Design review of the part built by this model. Coordinates are the model's own, in mm. A direction names the side the tool comes from. Coordinates: 2 decimals unless noted, no trailing zeros. Write each loop counter-clockwise with the first axis right and the second up, starting at its lowest first coordinate (ties: lowest second). Pieces come first, ordered by that corner, then holes. Notation, with made-up numbers: (42, -21.75) - (72, -21.75) arc R20 ccw to (72, -12.75) - close; hole circle Ø10 at (45.25, 79.5). An arc over 180 degrees is marked (long way). Use a Markdown table: item, result.
from build123d import *

# Parameters (mm, degrees)
ESQUISSE1_W             = 218
ESQUISSE1_H             = 80
ESQUISSE1_W_2           = 208
ESQUISSE1_H_2           = 70
BOSS_EXTRU_1_DEPTH      = 16.5
ESQUISSE2_W             = 15
ESQUISSE2_H             = 80
ESQUISSE2_R             = 3.25
BOSS_EXTRU_2_DEPTH      = 2.45
ESQUISSE3_W             = 22
ESQUISSE3_H             = 5
ENL_V_MAT_EXTRU_1_DEPTH = 16.5
ESQUISSE4_W             = 15
ESQUISSE4_H             = 70
ESQUISSE4_R             = 1.7
BOSS_EXTRU_3_DEPTH      = 3
CONG_1_R                = 20
ESQUISSE7_W             = 22
ESQUISSE7_H             = 5
BOSS_EXTRU_5_DEPTH      = 8
ESQUISSE8_W             = 52.75
ESQUISSE8_H             = 5
ESQUISSE8_W_2           = 24.75
ESQUISSE8_W_3           = 99.5
BOSS_EXTRU_6_DEPTH      = 2.45


with BuildPart() as part:
    # Esquisse1 → Boss.-Extru.1 (new body)
    with BuildSketch(Plane(origin=(0, 0, 0), x_dir=(1, 0, 0), z_dir=(0, 0.342020143, 0.939692621))):
        Rectangle(ESQUISSE1_W, ESQUISSE1_H)
        Rectangle(ESQUISSE1_W_2, ESQUISSE1_H_2, mode=Mode.SUBTRACT)
    extrude(amount=BOSS_EXTRU_1_DEPTH)

    # Esquisse2 → Boss.-Extru.2 (add)
    with BuildSketch(Plane(origin=(0, 0, 0), x_dir=(-1, 0, 0), z_dir=(0, -0.342020143, -0.939692621))):
        with Locations((-45.25, 0)):
            Rectangle(ESQUISSE2_W, ESQUISSE2_H)
        with Locations((-45.25, 29.75)):
            Circle(ESQUISSE2_R, mode=Mode.SUBTRACT)
        with Locations((-45.25, -29.75)):
            Circle(ESQUISSE2_R, mode=Mode.SUBTRACT)
        with Locations((69.25, 0)):
            Rectangle(ESQUISSE2_W, ESQUISSE2_H)
        with Locations((69.25, 29.75)):
            Circle(ESQUISSE2_R, mode=Mode.SUBTRACT)
        with Locations((69.25, -29.75)):
            Circle(ESQUISSE2_R, mode=Mode.SUBTRACT)
    extrude(amount=BOSS_EXTRU_2_DEPTH)

    # Esquisse3 → Enlèv. mat.-Extru.1 (cut)
    with BuildSketch(Plane(origin=(0, 5.643332365, 15.504928243), x_dir=(1, 0, 0), z_dir=(0, 0.342020143, 0.939692621))):
        with Locations((2, -37.5)):
            Rectangle(ESQUISSE3_W, ESQUISSE3_H)
    extrude(amount=-ENL_V_MAT_EXTRU_1_DEPTH, mode=Mode.SUBTRACT)

    # Esquisse4 → Boss.-Extru.3 (add)
    with BuildSketch(Plane(origin=(0, 0, 0), x_dir=(1, 0, 0), z_dir=(0, 0.342020143, 0.939692621))):
        with Locations((45.25, 0)):
            Rectangle(ESQUISSE4_W, ESQUISSE4_H)
        with Locations((45.25, -29.75)):
            Circle(ESQUISSE4_R, mode=Mode.SUBTRACT)
        with Locations((45.25, 29.75)):
            Circle(ESQUISSE4_R, mode=Mode.SUBTRACT)
        with Locations((-69.25, 0)):
            Rectangle(ESQUISSE4_W, ESQUISSE4_H)
        with Locations((-69.25, 29.75)):
            Circle(ESQUISSE4_R, mode=Mode.SUBTRACT)
        with Locations((-69.25, -29.75)):
            Circle(ESQUISSE4_R, mode=Mode.SUBTRACT)
    extrude(amount=BOSS_EXTRU_3_DEPTH)

    # Congé1
    cong_1_edges = [part.edges().sort_by_distance(p)[0] for p in [
        (52.75, -32.376211513, 13.380243948),
        (52.75, 33.402271942, -10.561166085),
        (-76.75, 33.402271942, -10.561166085),
        (-76.75, -32.376211513, 13.380243948),
    ]]
    fillet(cong_1_edges, radius=CONG_1_R)

    # Esquisse7 → Boss.-Extru.5 (add)
    with BuildSketch(Plane(origin=(0, 5.643332365, 15.504928243), x_dir=(1, 0, 0), z_dir=(0, 0.342020143, 0.939692621))):
        with Locations((2, -37.5)):
            Rectangle(ESQUISSE7_W, ESQUISSE7_H)
    extrude(amount=-BOSS_EXTRU_5_DEPTH)

    # Esquisse8 → Boss.-Extru.6 (add)
    with BuildSketch(Plane(origin=(0, 0, 0), x_dir=(-1, 0, 0), z_dir=(0, -0.342020143, -0.939692621))):
        with BuildLine():
            Line((76.75, -15), (76.75, -40))
            Line((76.75, -40), (109, -40))
            Line((109, -40), (109, 40))
            Line((109, 40), (76.75, 40))
            Line((76.75, 40), (76.75, 15))
            ThreePointArc((76.75, 15), (82.607864376, 29.142135624), (96.75, 35))
            Line((96.75, 35), (104, 35))
            Line((104, 35), (104, -35))
            Line((104, -35), (96.75, -35))
            ThreePointArc((96.75, -35), (82.607864376, -29.142135624), (76.75, -15))
        make_face()
        with BuildLine():
            Line((-52.75, 15), (-52.75, 40))
            Line((-52.75, 40), (-109, 40))
            Line((-109, 40), (-109, -40))
            Line((-109, -40), (-52.75, -40))
            Line((-52.75, -40), (-52.75, -15))
            ThreePointArc((-52.75, -15), (-58.607864376, -29.142135624), (-72.75, -35))
            Line((-72.75, -35), (-104, -35))
            Line((-104, -35), (-104, 35))
            Line((-104, 35), (-72.75, 35))
            ThreePointArc((-72.75, 35), (-58.607864376, 29.142135624), (-52.75, 15))
        make_face()
        with Locations((35.375, -37.5)):
            Rectangle(ESQUISSE8_W, ESQUISSE8_H)
        with Locations((-25.375, -37.5)):
            Rectangle(ESQUISSE8_W_2, ESQUISSE8_H)
        with Locations((12, 37.5)):
            Rectangle(ESQUISSE8_W_3, ESQUISSE8_H)
    extrude(amount=BOSS_EXTRU_6_DEPTH)


solid = part.part
(1) Take a section at C-C on z = 18. Write out the cut boundary in (x, y), and give its area (3 significant figures).
Determined:
| item | result |
|---|---|
| outline | (-109, -36.02) - (-9, -36.02) - (-9, -30.69) - (-104, -30.69) - (-104, -1.21) - (-109, -1.21) - close; (13, -36.02) - (109, -36.02) - (109, -1.21) - (104, -1.21) - (104, -30.69) - (13, -30.69) - close |
| area | 1,340 mm2 |
(2) Take a section at A-A on x = -41. Write out the cut boundary in (y, z), and give its area (4 significant figures).
Determined:
| item | result |
|---|---|
| outline | (-38.43, 11.38) - (-33.73, 9.67) - (-27.25, 27.48) - (-31.94, 29.19) - close; (32.05, -14.27) - (36.75, -15.98) - (43.23, 1.82) - (38.53, 3.53) - close |
| area | 189.5 mm2 |
(3) Draft analysis for pull direction Z (two halves, no side actions). For faces 1 (the flat face through (-1.46, -29.72, 20.68)), 2 (the flat face through (-76.75, 0, 0)), 3 (the flat face through (1.456, 36.057, -3.266)), state which applies: +Z half, -Z half, draft (parallel to the pull), parting line (faces both ways), or undercut.
Determined:
| item | result |
|---|---|
| face 1 | undercut |
| face 2 | draft |
| face 3 | +Z half |
(4) Take a section at B-B on y = 11. Write out the cut boundary in (x, z), and give its area (3 significant figures).
Determined:
| item | result |
|---|---|
| outline | (-109, -6.61) - (-104, -6.61) - (-104, 13.56) - (-109, 13.56) - close; (-76.75, -6.61) - (-61.75, -6.61) - (-61.75, -0.81) - (-76.75, -0.81) - close; (37.75, -6.61) - (52.75, -6.61) - (52.75, -0.81) - (37.75, -0.81) - close; (104, -6.61) - (109, -6.61) - (109, 13.56) - (104, 13.56) - close |
| area | 376 mm2 |
(5) Take a section at D-D on x = 0. Write out the cut boundary in (y, z).
Determined:
| item | result |
|---|---|
| outline | (-34.68, 21.67) - (-29.98, 19.96) - (-27.25, 27.48) - (-31.94, 29.19) - close; (32.05, -14.27) - (36.75, -15.98) - (43.23, 1.82) - (38.53, 3.53) - close |
(6) For pin 1 (8 mm diameter, centred on x = 80.5, z = 22.5, fed in from +Y); pin 2 (5 mm diameter, centred on x = 41.5, y = -22.5, fed in from +Z); pin 3 (3 mm diameter, centred on x = -63, z = 2.5, fed in from +Y), all flat-tipped, find the tip position at first contact; note any pin that passes through.
Determined:
| item | result |
|---|---|
| pin 1 | y = -27.6 |
| pin 2 | z = 12.29 |
| pin 3 | y = 43.23 |
(7) Machinability: for faces 4 (the flat face through (0.51, 35.53, -15.54)), 5 (the flat face through (46.649, 26.641, -9.697)), 6 (the flat face through (1.8, -32.3, 20.8)), 7 (the flat face through (52.75, 0, 0)), which of the approach directions +Z, -Z, +X, -X, +Y, -Y give a long, thin tool a straight path to every point of the face, cutting with its end or side? Answer none if there is none.
Determined:
| item | result |
|---|---|
| face 4 | -Z, +X, -X, -Y |
| face 5 | none |
| face 6 | -Z, -Y |
| face 7 | +Z, -Z |
(8) For L1, parallel to X at y = 25, z = -11.5; L2, parallel to X at y = -8, z = 11; L3, parallel to X at y = 31, z = -13, list the stretches that pass through material, from the lowest coordinate up. Write a range as from..to.
Determined:
| item | result |
|---|---|
| L1 | -109..-104, -81.08..-71.52, -66.98..-61.75, 37.75..42.98, 47.52..57.08, 104..109 |
| L2 | -109..-104, 104..109 |
| L3 | -109..-104, -89.34..-61.75, 37.75..65.34, 104..109 |
